```python
from build123d import *

# Parameters (mm, degrees)
BOSS_EXTRUDE1_DEPTH  = 1
PCB_HOLDER_52_R      = 4.5
BOSS_EXTRUDE2_DEPTH  = 1
BOSS_EXTRUDE3_DEPTH  = 2
PCB_HOLDER_57_W      = 17.5
PCB_HOLDER_57_H      = 0.75
BOSS_EXTRUDE7_DEPTH  = 5
SKETCH6_W            = 9.5
SKETCH6_H            = 1.75
BOSS_EXTRUDE9_DEPTH  = 1.75
CUT_EXTRUDE7_DEPTH   = 0.75
PCB_HOLDER_58_W      = 2.5
PCB_HOLDER_58_H      = 1
PCB_HOLDER_58_H_2    = 0.75
BOSS_EXTRUDE10_DEPTH = 11.25
SKETCH10_W           = 2.5
SKETCH10_H           = 2
BOSS_EXTRUDE11_DEPTH = 2
CUT_EXTRUDE8_DEPTH   = 15
CUT_EXTRUDE12_DEPTH  = 9.5
CUT_EXTRUDE17_DEPTH  = 1
BOSS_EXTRUDE12_START = 3
BOSS_EXTRUDE12_DEPTH = 3
SKETCH13_4_W         = 11
SKETCH13_4_H         = 1
CUT_EXTRUDE18_DEPTH  = 3


with BuildPart() as part:
    # PCB holder → Boss-Extrude1 (new body)
    with BuildSketch(Plane(origin=(0, 0, 0), x_dir=(1, 0, 0), z_dir=(0, 1, 0))):
        with BuildLine():
            Line((9, 21.5), (-9, 21.5))
            ThreePointArc((-9, 21.5), (-9.707106781, 21.207106781), (-10, 20.5))
            Line((-10, 20.5), (-10, -14.5))
            ThreePointArc((-10, -14.5), (-9.707106781, -15.207106781), (-9, -15.5))
            Line((-9, -15.5), (9, -15.5))
            ThreePointArc((9, -15.5), (9.707106781, -15.207106781), (10, -14.5))
            Line((10, -14.5), (10, 20.5))
            ThreePointArc((10, 20.5), (9.707106781, 21.207106781), (9, 21.5))
        make_face()
        with BuildLine():
            Line((9.25, 14.25), (9.25, -14.25))
            ThreePointArc((9.25, -14.25), (9.103553391, -14.603553391), (8.75, -14.75))
            Line((8.75, -14.75), (-8.75, -14.75))
            ThreePointArc((-8.75, -14.75), (-9.103553391, -14.603553391), (-9.25, -14.25))
            Line((-9.25, -14.25), (-9.25, 14.25))
            ThreePointArc((-9.25, 14.25), (-9.103553391, 14.603553391), (-8.75, 14.75))
            Line((-8.75, 14.75), (8.75, 14.75))
            ThreePointArc((8.75, 14.75), (9.103553391, 14.603553391), (9.25, 14.25))
        make_face(mode=Mode.SUBTRACT)
    extrude(amount=BOSS_EXTRUDE1_DEPTH)

    # PCB holder<52> → Boss-Extrude2 (add)
    with BuildSketch(Plane(origin=(0, 0, 0), x_dir=(1, 0, 0), z_dir=(0, 1, 0))):
        with BuildLine():
            Line((-9.25, 14.25), (-9.25, -14.25))
            ThreePointArc((-9.25, -14.25), (-9.103553391, -14.603553391), (-8.75, -14.75))
            Line((-8.75, -14.75), (8.75, -14.75))
            ThreePointArc((8.75, -14.75), (9.103553391, -14.603553391), (9.25, -14.25))
            Line((9.25, -14.25), (9.25, 14.25))
            ThreePointArc((9.25, 14.25), (9.103553391, 14.603553391), (8.75, 14.75))
            Line((8.75, 14.75), (-8.75, 14.75))
            ThreePointArc((-8.75, 14.75), (-9.103553391, 14.603553391), (-9.25, 14.25))
        make_face()
        with Locations(Location((0, -5, 0), (0, 0, 270))):
            Circle(PCB_HOLDER_52_R, mode=Mode.SUBTRACT)
        with Locations(Location((0, 5, 0), (0, 0, 270))):
            Circle(PCB_HOLDER_52_R, mode=Mode.SUBTRACT)
    extrude(amount=BOSS_EXTRUDE2_DEPTH)

    # PCB holder<55> → Boss-Extrude3 (add)
    with BuildSketch(Plane(origin=(0, 0, 0), x_dir=(1, 0, 0), z_dir=(0, 1, 0))):
        with BuildLine():
            Line((8.75, 15.5), (8.75, 14.75))
            ThreePointArc((8.75, 14.75), (9.103553391, 14.603553391), (9.25, 14.25))
            Line((9.25, 14.25), (9.25, -14.25))
            ThreePointArc((9.25, -14.25), (9.103553391, -14.603553391), (8.75, -14.75))
            Line((8.75, -14.75), (7.5, -14.75))
            Line((7.5, -14.75), (7.5, -15.5))
            Line((7.5, -15.5), (9, -15.5))
            ThreePointArc((9, -15.5), (9.707106781, -15.207106781), (10, -14.5))
            Line((10, -14.5), (10, 20.5))
            ThreePointArc((10, 20.5), (9.707106781, 21.207106781), (9, 21.5))
            Line((9, 21.5), (-9, 21.5))
            ThreePointArc((-9, 21.5), (-9.707106781, 21.207106781), (-10, 20.5))
            Line((-10, 20.5), (-10, -14.5))
            ThreePointArc((-10, -14.5), (-9.707106781, -15.207106781), (-9, -15.5))
            Line((-9, -15.5), (-7.5, -15.5))
            Line((-7.5, -15.5), (-7.5, -14.75))
            Line((-7.5, -14.75), (-8.75, -14.75))
            ThreePointArc((-8.75, -14.75), (-9.103553391, -14.603553391), (-9.25, -14.25))
            Line((-9.25, -14.25), (-9.25, 14.25))
            ThreePointArc((-9.25, 14.25), (-9.103553391, 14.603553391), (-8.75, 14.75))
            Line((-8.75, 14.75), (-8.75, 15.5))
            Line((-8.75, 15.5), (8.75, 15.5))
        make_face()
    extrude(amount=BOSS_EXTRUDE3_DEPTH)

    # PCB holder<57> → Boss-Extrude7 (add)
    with BuildSketch(Plane(origin=(0, 0, 0), x_dir=(1, 0, 0), z_dir=(0, 1, 0))):
        with Locations((0, 15.125)):
            Rectangle(PCB_HOLDER_57_W, PCB_HOLDER_57_H)
    extrude(amount=BOSS_EXTRUDE7_DEPTH)

    # Sketch6 → Boss-Extrude9 (add)
    with BuildSketch(Plane.XY.offset(-14.75)):
        with Locations((0, 4.125)):
            Rectangle(SKETCH6_W, SKETCH6_H)
    extrude(amount=BOSS_EXTRUDE9_DEPTH)

    # Sketch8 → Cut-Extrude7 (cut)
    with BuildSketch(Plane.XY.offset(-14.75)):
        Polygon((4.75, 5), (8.75, 2), (8.75, 5), align=None)
        Polygon((-4.75, 5), (-8.75, 2), (-8.75, 5), align=None)
    extrude(amount=-CUT_EXTRUDE7_DEPTH, mode=Mode.SUBTRACT)

    # PCB holder<58> → Boss-Extrude10 (add)
    with BuildSketch(Plane(origin=(0, 0, 0), x_dir=(1, 0, 0), z_dir=(0, 1, 0))):
        with Locations((-6.25, -16)):
            Rectangle(PCB_HOLDER_58_W, PCB_HOLDER_58_H)
        with Locations((-6.25, -15.125)):
            Rectangle(PCB_HOLDER_58_W, PCB_HOLDER_58_H_2)
        with Locations((6.25, -16)):
            Rectangle(PCB_HOLDER_58_W, PCB_HOLDER_58_H)
        with Locations((6.25, -15.125)):
            Rectangle(PCB_HOLDER_58_W, PCB_HOLDER_58_H_2)
    extrude(amount=BOSS_EXTRUDE10_DEPTH)

    # Sketch10 → Boss-Extrude11 (add)
    with BuildSketch(Plane(origin=(0, 0, 14.75), x_dir=(-1, 0, 0), z_dir=(0, 0, -1))):
        with Locations((-6.25, 10.25)):
            Rectangle(SKETCH10_W, SKETCH10_H)
        with Locations((6.25, 10.25)):
            Rectangle(SKETCH10_W, SKETCH10_H)
    extrude(amount=BOSS_EXTRUDE11_DEPTH)

    # Sketch11 → Cut-Extrude8 (cut)
    with BuildSketch(Plane(origin=(7.5, 0, 0), x_dir=(0, 0, -1), z_dir=(1, 0, 0))):
        Polygon((-14.75, 11.25), (-12.75, 9.25), (-12.75, 11.25), align=None)
    extrude(amount=-CUT_EXTRUDE8_DEPTH, mode=Mode.SUBTRACT)

    # Sketch7 → Cut-Extrude12 (cut)
    with BuildSketch(Plane(origin=(4.75, 0, 0), x_dir=(0, 0, -1), z_dir=(1, 0, 0))):
        Polygon((13, 3.25), (14.75, 5), (13, 5), align=None)
    extrude(amount=-CUT_EXTRUDE12_DEPTH, mode=Mode.SUBTRACT)

    # Sketch13 → Cut-Extrude17 (cut)
    with BuildSketch(Plane(origin=(0, 2, 0), x_dir=(1, 0, 0), z_dir=(0, 1, 0))):
        with BuildLine():
            Line((8.75, 20.75), (-8.75, 20.75))
            ThreePointArc((-8.75, 20.75), (-9.103553391, 20.603553391), (-9.25, 20.25))
            Line((-9.25, 20.25), (-9.25, 16))
            ThreePointArc((-9.25, 16), (-9.103553391, 15.646446609), (-8.75, 15.5))
            Line((-8.75, 15.5), (-2.197469764, 15.5))
            ThreePointArc((-2.197469764, 15.5), (0, 17.697469764), (2.197469764, 15.5))
            Line((2.197469764, 15.5), (8.75, 15.5))
            ThreePointArc((8.75, 15.5), (9.103553391, 15.646446609), (9.25, 16))
            Line((9.25, 16), (9.25, 20.25))
            ThreePointArc((9.25, 20.25), (9.103553391, 20.603553391), (8.75, 20.75))
        make_face()
    extrude(amount=-CUT_EXTRUDE17_DEPTH, mode=Mode.SUBTRACT)

    # Sketch13<3> → Boss-Extrude12 (add)
    with BuildSketch(Plane(origin=(0, 2, 0), x_dir=(1, 0, 0), z_dir=(0, 1, 0)).offset(BOSS_EXTRUDE12_START)):
        with BuildLine():
            ThreePointArc((2.197469764, 15.5), (0, 17.697469764), (-2.197469764, 15.5))
            Line((-2.197469764, 15.5), (2.197469764, 15.5))
        make_face()
    extrude(amount=-BOSS_EXTRUDE12_DEPTH)

    # Sketch13<4> → Cut-Extrude18 (cut)
    with BuildSketch(Plane(origin=(0, 2, 0), x_dir=(1, 0, 0), z_dir=(0, 1, 0))):
        with Locations((2.5, 19)):
            Rectangle(SKETCH13_4_W, SKETCH13_4_H)
    extrude(amount=-CUT_EXTRUDE18_DEPTH, mode=Mode.SUBTRACT)


solid = part.part
```
Work out the finished part from the listing and answer in its coordinate system (mm). A direction names the side the tool comes from. Round coordinates to 2 decimals unless told otherwise and drop trailing zeros. Loops run counter-clockwise (first coordinate to the right, second up) from the corner with the lowest first, then second, coordinate; pieces in that order, holes last. Notation, with made-up numbers: (60, 68.25) -> (118, 68.25) arc R24 ccw to (118, 92.25) -> close; hole circle Ø9 at (81, 74). An arc over 180 degrees is marked (long way). Write each question's results on one line, items separated by ' | '. Start each with the question number.
1. A tool of negligible diameter and unlimited length cuts with its end or side. For faces 1 (the face through (8, 1, 15.5)), 2 (the face through (8, 0.5, -19)), 3 (the face through (-0.1, 0.5, 15.5)), 4 (the face through (6, 9.25, 14)), from which of +Z, -Z, +X, -X, +Y, -Y can it reach the whole face along a straight path? Write none if from no direction.
2. Section B-B (z = -5) is taken. Determine the outline of the cut face in (x, y).
3. Section D-D (y = 2.5) is taken. Determine the outline of the cut face in (x, z).
4. Given pin 1 Ø4 at (x, z) = (2, 7.5) entering from +Y; pin 2 Ø0.5 at (x, y) = (4, 0.5) entering from +Z; pin 3 Ø0.5 at (y, z) = (4.5, -14) entering from -X, each flat-ended and moving along its own axis, determine where each tip first touches the part or whether it passes through.
5. Section C-C (y = 8.5) is taken. Determine the outline of the cut face in (x, z).
6. Find the intervals of material crossed by probe 1 along X at (y, z) = (0.5, -5); probe 2 along Y at (x, z) = (-5.5, 4.5); probe 3 along Z at (x, y) = (6, 8.25), in increasing order. Write a range as from..to.
7. For a pull along Y with two mould halves and no side action, classify faces 5 (the face through (6, 5, 14.75)), 6 (the face through (9.715, 0.986, -21.199)), 7 (the face through (0.07, 4.11, -13.86)) as +Y half, -Y half, draft (parallel to the pull), parting line (faces both ways), or undercut.
8. Section A-A (x = 0) is taken. Determine the outline of the cut face in (y, z).
Evaluation:
1) face 1: +Z, +X, +Y, -Y | face 2: +Y, -Y | face 3: +Z, +Y, -Y | face 4: -Z, +X, -X
2) outline: (-10, 0) -> (-4.5, 0) -> (-4.5, 1) -> (-9.25, 1) -> (-9.25, 2) -> (-10, 2) -> close; (4.5, 0) -> (10, 0) -> (10, 2) -> (9.25, 2) -> (9.25, 1) -> (4.5, 1) -> close
3) outline: (-8.08, -15.5) -> (-2.2, -15.5) arc R2.2 ccw to (2.2, -15.5) -> (8.08, -15.5) -> (8.08, -14.75) -> (-8.08, -14.75) -> close; (-7.5, 14.75) -> (-5, 14.75) -> (-5, 16.5) -> (-7.5, 16.5) -> close; (5, 14.75) -> (7.5, 14.75) -> (7.5, 16.5) -> (5, 16.5) -> close
4) pin 1: stops at y = 1 | pin 2: stops at z = 15.5 | pin 3: stops at x = -4.75
5) outline: (-7.5, 14.75) -> (-5, 14.75) -> (-5, 16.5) -> (-7.5, 16.5) -> close; (5, 14.75) -> (7.5, 14.75) -> (7.5, 16.5) -> (5, 16.5) -> close
6) probe 1: x = -10..-4.5, 4.5..10 | probe 2: y = 0..1 | probe 3: z = 14.75..16.5
7) face 5: undercut | face 6: draft | face 7: +Y half
8) outline: (0, -21.5) -> (2, -21.5) -> (2, -20.75) -> (1, -20.75) -> (1, -19.5) -> (0, -19.5) -> close; (0, -18.5) -> (1, -18.5) -> (1, -17.7) -> (5, -17.7) -> (5, -14.75) -> (3.25, -13) -> (3.25, -14.75) -> (1, -14.75) -> (1, -9.5) -> (0, -9.5) -> close; (0, -0.5) -> (1, -0.5) -> (1, 0.5) -> (0, 0.5) -> close; (0, 9.5) -> (1, 9.5) -> (1, 15.5) -> (0, 15.5) -> close
